from build123d import *

# Parameters (mm, degrees)
F0_R     = 6
F2_DEPTH = 25
F3_DEPTH = 25
F4_R     = 1


with BuildPart() as f2:
    # F0 (on Top) → F2 (new body)
    with BuildSketch(Plane.XY):
        Circle(F0_R)
    extrude(amount=F2_DEPTH)

    # F1 (on Top) → F3 (cut)
    with BuildSketch(Plane.XY):
        with BuildLine():
            Line((-2.05, 1.341641), (-2.05, -1.341641))
            ThreePointArc((-2.05, -1.341641), (2.45, 0), (-2.05, 1.341641))
        make_face()
    extrude(amount=F3_DEPTH, mode=Mode.SUBTRACT)

    # F4
    f4_edges = [f2.edges().sort_by_distance(p)[0] for p in [
        (-6, 0, 25),
        (-6, 0, 0),
    ]]
    fillet(f4_edges, radius=F4_R)


solid = f2.part
Work out the finished part from the listing and answer in its coordinate system (mm). A direction names the side the tool comes from. Round coordinates to 2 decimals unless told otherwise and drop trailing zeros. Loops run counter-clockwise (first coordinate to the right, second up) from the corner with the lowest first, then second, coordinate; pieces in that order, holes last. Notation, with made-up numbers: (44, 28.25) - (92, 28.25) arc R19 ccw to (92, 43.25) - close; hole circle Ø10 at (-18, -27.75). An arc over 180 degrees is marked (long way). One line per item, written item: value.
Q1. Find section A-A on x = 0. Give the vertices of the cut face in (y, z), and give its area (3 significant figures).
Check values:
outline: (-6, 1) arc R1 ccw to (-5, 0) - (-2.45, 0) - (-2.45, 25) - (-5, 25) arc R1 ccw to (-6, 24) - close; (2.45, 0) - (5, 0) arc R1 ccw to (6, 1) - (6, 24) arc R1 ccw to (5, 25) - (2.45, 25) - close
area: 177 mm2
Q2. The mould has two halves that part along Y. Classify faces 1 (the flat face through (-2.3, 0.1, 0)), 2 (the cylindrical face through (2.45, -0.09, 12.32)), 3 (the cylindrical face through (-6, 0, 12)): +Y half, -Y half, draft (parallel to the pull), parting line (faces both ways), or undercut.
Check values:
face 1: draft
face 2: undercut
face 3: parting line
Q3. Straight lines are drawn through the part: probe 1 along Y at (x, z) = (0, 15); probe 2 along X at (y, z) = (0.5, 14.5); probe 3 along Z at (x, y) = (-1, 5). For each, find the intervals that lie inside material, in ascending order.
Check values:
probe 1: -6 to -2.45, 2.45 to 6
probe 2: -5.98 to -2.05, 2.4 to 5.98
probe 3: 0 to 25
Q4. Find section C-C on z = 4.75. Give the vertices of the cut face in (x, y), and give its area (3 significant figures).
Check values:
outline: circle Ø12 at (0, 0); hole (-2.05, -1.34) arc R2.45 ccw (long way) to (-2.05, 1.34) - close
area: 95.0 mm2
Q5. Each of these flat-tipped pins is pushed along its axis until it touches: pin 1 Ø3 at (x, z) = (3.5, 11) entering from +Y; pin 2 Ø1.5 at (y, z) = (-2.5, 20) entering from -X; pin 3 Ø1.5 at (y, z) = (-2, 19) entering from +X. Where does it stop, or does it pass through?
Check values:
pin 1: y = 5.66
pin 2: x = -5.74
pin 3: x = 5.87
Q6. For faces 4 (the flat face through (-2.05, 0, 12)), 5 (the flat face through (-2.3, 0.1, 25)), determine the directions among +Z, -Z, +X, -X, +Y, -Y from which every point of the face is accessible in a straight line to the end or side of a thin tool.
Check values:
face 4: +Z, -Z
face 5: +Z, +X, -X, +Y, -Y
Q7. Find section B-B on y = 0. Give the vertices of the cut face in (x, z).
Check values:
outline: (-6, 1) arc R1 ccw to (-5, 0) - (-2.05, 0) - (-2.05, 25) - (-5, 25) arc R1 ccw to (-6, 24) - close; (2.45, 0) - (5, 0) arc R1 ccw to (6, 1) - (6, 24) arc R1 ccw to (5, 25) - (2.45, 25) - close
